Source: CAD feature listing. Evaluate the final solid. Frame: model axes, mm. A direction names the side the tool comes from. Give positions to 0.01 mm unless a question says otherwise; leave off trailing zeros. Loops run counter-clockwise (first coordinate to the right, second up) from the corner with the lowest first, then second, coordinate; pieces in that order, holes last. Notation, with made-up numbers: M -19,16 L 33,16 A31 cw 33,51 Z; hole C 71.5,75 d2. An arc over 180 degrees is marked long. Put each result on its own line as item: value.
from build123d import *

# Parameters (mm, degrees)
ESQUISSE1_W             = 60
ESQUISSE1_H             = 55
BOSS_EXTRU_1_DEPTH      = 1.5
CONG_1_R                = 2
ESQUISSE2_R             = 1.5
ENL_V_MAT_EXTRU_1_DEPTH = 1.5
ESQUISSE3_W             = 16
ESQUISSE3_H             = 23
BOSS_EXTRU_2_DEPTH      = 25


with BuildPart() as part:
    # Esquisse1 → Boss.-Extru.1 (new body)
    with BuildSketch(Plane.XY):
        with Locations((30, 27.5)):
            Rectangle(ESQUISSE1_W, ESQUISSE1_H)
    extrude(amount=BOSS_EXTRU_1_DEPTH)

    # Congé1
    cong_1_edges = [part.edges().sort_by_distance(p)[0] for p in [
        (0, 55, 0.75),
        (60, 55, 0.75),
        (60, 0, 0.75),
        (0, 0, 0.75),
    ]]
    fillet(cong_1_edges, radius=CONG_1_R)

    # Esquisse2 → Enlèv. mat.-Extru.1 (cut)
    with BuildSketch(Plane(origin=(0, 0, 0), x_dir=(-1, 0, 0), z_dir=(0, 0, -1))):
        with Locations((-5, 5)):
            Circle(ESQUISSE2_R)
        with Locations((-5, 50)):
            Circle(ESQUISSE2_R)
        with Locations((-55, 50)):
            Circle(ESQUISSE2_R)
        with Locations((-55, 5)):
            Circle(ESQUISSE2_R)
    extrude(amount=-ENL_V_MAT_EXTRU_1_DEPTH, mode=Mode.SUBTRACT)

    # Esquisse3 → Boss.-Extru.2 (add)
    with BuildSketch(Plane(origin=(0, 0, 0), x_dir=(-1, 0, 0), z_dir=(0, 0, -1))):
        with Locations((-35, 26.5)):
            Rectangle(ESQUISSE3_W, ESQUISSE3_H)
    extrude(amount=BOSS_EXTRU_2_DEPTH)


solid = part.part
1. Draft query along Y for faces 4 (the flat face through (23, 28, 0)), 5 (the cylindrical face through (59.4, 0.57, 0.76)), 6 (the cylindrical face through (5.325, 48.536, 0.74)). Return one class per face: pulls with the +Y half, pulls with the -Y half, needs draft (parallel to the pull), parting line crosses it, or undercut.
Found:
face 4: needs draft
face 5: pulls with the -Y half
face 6: undercut
2. Section query A-A (y = 28). Output: boundary loops of the cut face in (x, z).
Found:
outline: M 0,0 L 27,0 L 27,-25 L 43,-25 L 43,0 L 60,0 L 60,1.5 L 0,1.5 Z
3. Access query for faces 1 (the flat face through (27, 26, -12)), 2 (the flat face through (43, 26, -12)), 3 (the flat face through (35, 15, -12)). Directions: +Z, -Z, +X, -X, +Y, -Y. A direction counts if a zero-diameter tool reaches every point of the face in a straight line with its end or side. Return the directions, or none.
Found:
face 1: -Z, -X, +Y, -Y
face 2: -Z, +X, +Y, -Y
face 3: -Z, +X, -X, -Y
4. Material intervals for line 1 (Y direction, x = 55, z = 0.5); line 2 (Z direction, x = 13, y = 46); line 3 (X direction, y = 30, z = -5), sorted ascending. Write a range as from..to.
Found:
line 1: 0..3.5, 6.5..48.5, 51.5..55
line 2: 0..1.5
line 3: 27..43
5. Section query C-C (y = 5). Output: boundary loops of the cut face in (x, z), plus the area to 3 significant figures.
Found:
outline: M 0,0 L 3.5,0 L 3.5,1.5 L 0,1.5 Z; M 6.5,0 L 53.5,0 L 53.5,1.5 L 6.5,1.5 Z; M 56.5,0 L 60,0 L 60,1.5 L 56.5,1.5 Z
area: 81.0 mm^2
6. Section query B-B (x = 55). Output: boundary loops of the cut face in (y, z).
Found:
outline: M 0,0 L 3.5,0 L 3.5,1.5 L 0,1.5 Z; M 6.5,0 L 48.5,0 L 48.5,1.5 L 6.5,1.5 Z; M 51.5,0 L 55,0 L 55,1.5 L 51.5,1.5 Z
7. Contact query for flat-ended pins moving along their axis: P1, Ø5, axis at x = 33, z = -8.5, coming from the +Y side; P2, Ø7, axis at y = 32, z = -14, coming from the +X side; P3, Ø5, axis at x = 33, z = -11, coming from the -Y side; P4, Ø4, axis at x = 55, y = 50, coming from the +Z side. Output: stop coordinate, or through.
Found:
P1: y = 38
P2: x = 43
P3: y = 15
P4: z = 1.5
8. Section query D-D (x = 35.5). Output: boundary loops of the cut face in (y, z).
Found:
outline: M 0,0 L 15,0 L 15,-25 L 38,-25 L 38,0 L 55,0 L 55,1.5 L 0,1.5 Z
